from build123d import *

# Parameters (mm, degrees)
LEG_AND_PAD_DEPTH          = 13
SCREW_HEAD_RELIEF_SKETCH_W = 14
SCREW_HEAD_RELIEF_SKETCH_H = 6
SCREW_HEAD_RELIEF_DEPTH    = 2.35
M6_SLOT_MIDDLE_DEPTH       = 3.5
SCREW_HOLES_SKETCH_R       = 1.95
SCREW_HOLES_DEPTH          = 4.5


with BuildPart() as part:
    # leg and pad sketch → leg and pad (new, symmetric)
    with BuildSketch(Plane(origin=(0, -20.7, 0), x_dir=(1, 0, 0), z_dir=(0, 1, 0))):
        Polygon((0.551289683, 30.332713936), (0.367250577, 30.819395741), (0.028023026, 31.213926146), (-0.425575667, 31.468833575), (-0.938966578, 31.553446481), (-1.450376329, 31.457583879), (-1.898269923, 31.192780366), (-2.228754897, 30.790898227), (-2.402065893, 30.30029363), (-2.397349395, 29.779998208), (-2.215172912, 29.292616119), (-1.877456693, 28.896791249), (-1.424836191, 28.640150931), (-0.91177263, 28.55357522), (-0.4, 28.647481273), (-0.4, -9.98), (-1.92, -11.5), (-1.92, -31.37), (-8.92, -31.37), (-8.92, 32.792642706), (27.204821487, 54.594667874), (30.821788068, 48.601542416), align=None)
    extrude(amount=LEG_AND_PAD_DEPTH, both=True)

    # screw head relief sketch → screw head relief (cut, symmetric)
    with BuildSketch(Plane(origin=(-1.35, 0, 0), x_dir=(0, 0, -1), z_dir=(1, 0, 0))):
        with Locations((16.4, -9.7)):
            Rectangle(SCREW_HEAD_RELIEF_SKETCH_W, SCREW_HEAD_RELIEF_SKETCH_H)
    extrude(amount=SCREW_HEAD_RELIEF_DEPTH, both=True, mode=Mode.SUBTRACT)

    # insert flange relief sketch → insert flange relief (revolve, cut)
    with BuildSketch(Plane(origin=(0, -20.7, 0), x_dir=(1, 0, 0), z_dir=(0, 1, 0)), mode=Mode.PRIVATE) as insert_flange_relief_sk:
        Polygon((18.324853729, 39.891397061), (17.03307995, 42.03179901), (9.755713323, 37.639768162), (11.047487102, 35.499366213), align=None)
    revolve(insert_flange_relief_sk.sketch.rotate(Axis((18.324853729, -20.7, -39.891397061), (-0.5167095115681243, 0, -0.8561607796757748)), 180), axis=Axis((18.324853729, -20.7, -39.891397061), (-0.5167095115681243, 0, -0.8561607796757748)), mode=Mode.SUBTRACT)

    # M6 slot end 1 sketch → M6 slot end 1 (revolve, cut)
    with BuildSketch(Plane(origin=(0, -20.7, 0), x_dir=(1, 0, 0), z_dir=(0, 1, 0)), mode=Mode.PRIVATE) as m6_slot_end_1_sk:
        Polygon((20.893336068, 41.441525596), (16.242950464, 49.146972613), (13.246387735, 47.338489322), (17.896773339, 39.633042305), align=None)
    revolve(m6_slot_end_1_sk.sketch.rotate(Axis((20.893336068, -20.7, -41.441525596), (-0.5167095115681233, 0, -0.8561607796757753)), 180), axis=Axis((20.893336068, -20.7, -41.441525596), (-0.5167095115681233, 0, -0.8561607796757753)), mode=Mode.SUBTRACT)

    # M6 slot end 2 sketch → M6 slot end 2 (revolve, cut)
    with BuildSketch(Plane(origin=(0, -20.7, 0), x_dir=(1, 0, 0), z_dir=(0, 1, 0))):
        Polygon((15.75637139, 38.341268526), (11.105985786, 46.046715543), (8.109423057, 44.238232253), (12.759808661, 36.532785236), align=None)
    revolve(axis=Axis((15.75637139, -20.7, -38.341268526), (-0.5167095115681234, 0, -0.8561607796757752)), mode=Mode.SUBTRACT)

    # M6 slot middle sketch → M6 slot middle (cut, symmetric)
    with BuildSketch(Plane(origin=(0, -20.7, 0), x_dir=(1, 0, 0), z_dir=(0, 1, 0))):
        Polygon((15.75637139, 38.341268526), (20.893336068, 41.441525596), (16.242950464, 49.146972613), (11.105985786, 46.046715543), align=None)
    extrude(amount=M6_SLOT_MIDDLE_DEPTH, both=True, mode=Mode.SUBTRACT)

    # screw holes sketch → screw holes (cut, symmetric)
    with BuildSketch(Plane(origin=(-5.42, 0, 0), x_dir=(0, 0, -1), z_dir=(1, 0, 0))):
        with Locations((-20.375, -28.7)):
            Circle(SCREW_HOLES_SKETCH_R)
        with Locations((-20.375, -12.7)):
            Circle(SCREW_HOLES_SKETCH_R)
    extrude(amount=SCREW_HOLES_DEPTH, both=True, mode=Mode.SUBTRACT)


solid = part.part
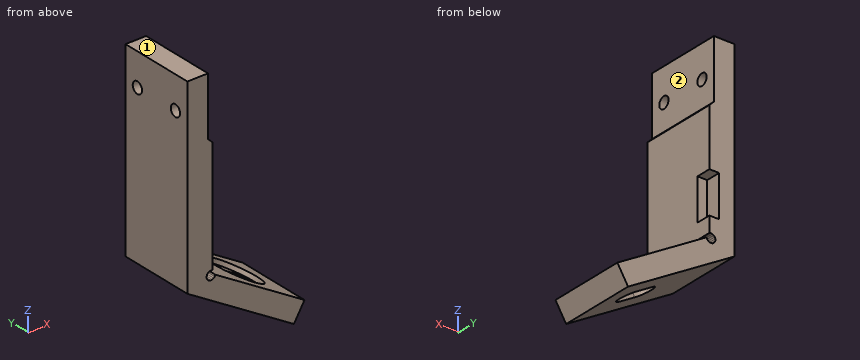
Build history of the part. All positions in model axes, mm. Face numbers are marked on the shaded views. A direction names the side the tool comes from. Round coordinates to 2 decimals unless told otherwise and drop trailing zeros. Loops run counter-clockwise (first coordinate to the right, second up) from the corner with the lowest first, then second, coordinate; pieces in that order, holes last. Notation, with made-up numbers: (51, 63.25) -> (83, 63.25) arc R33 ccw to (83, 102.25) -> close; hole circle Ø1 at (-9, -6). An arc over 180 degrees is marked (long way). One line per item, written item: value. Start each with the question number.
Q1. 3-axis set-ups, long thin cutter, end or side, ignore diameter. For the marked faces 1 and 2: which of +Z, -Z, +X, -X, +Y, -Y reach the whole face in a straight line?
Q2. Probe line 1 along Z through (x, y) = (-1, -11); line 2 along Z through (x, y) = (-2.85, -28.7) (3 decimals); line 3 along X through (y, z) = (-28.5, -5.5). List the from-to ranges inside material, lowest first.
Q3. Drop flat-ended pins along their axis: pin 1 Ø5 at (x, z) = (4.5, -32) entering from -Y; pin 2 Ø10 at (y, z) = (-19.5, 21.5) entering from +X; pin 3 Ø1.6 at (x, z) = (-2, -16.5) entering from +Y; pin 4 Ø8 at (y, z) = (-23.5, -7.5) entering from +X. Give the stop position or say it passes through.
Q4. Cut at A-A on y = -31.5. List the corners of the cut face in (x, z).
Q5. Cut at B-B on z = -25. List the corners of the cut face in (x, y).
Computed:
1. face 1: +Z, +X, -X, +Y, -Y
1. face 2: +Z, +X, +Y, -Y
2. line 1: -37.57 to -31.54, -28.57 to -23.4, -9.4 to 10.58
2. line 2: -36.456 to 18.425, 22.325 to 31.37
2. line 3: -8.92 to -0.4
3. pin 1: y = -33.7
3. pin 2: x = -1.92
3. pin 3: y = -12.7
3. pin 4: x = -0.4
4. outline: (-8.92, -32.79) -> (27.2, -54.59) -> (30.82, -48.6) -> (0.55, -30.33) -> (0.37, -30.82) -> (0.03, -31.21) -> (-0.43, -31.47) -> (-0.94, -31.55) -> (-1.45, -31.46) -> (-1.9, -31.19) -> (-2.23, -30.79) -> (-2.4, -30.3) -> (-2.4, -29.78) -> (-2.22, -29.29) -> (-1.88, -28.9) -> (-1.42, -28.64) -> (-0.91, -28.55) -> (-0.4, -28.65) -> (-0.4, 9.98) -> (-1.92, 11.5) -> (-1.92, 31.37) -> (-8.92, 31.37) -> close
5. outline: (-8.92, -33.7) -> (-0.4, -33.7) -> (-0.4, -7.7) -> (-8.92, -7.7) -> close
